Autodesk Inventor part; units mm, degrees
ref_plane "YZ Plane" through (0, 0, 0) normal (1, 0, 0) x (0, 1, 0)
ref_plane "XZ Plane" through (0, 0, 0) normal (0, 1, 0) x (-1, 0, 0)
ref_plane "XY Plane" through (0, 0, 0) normal (0, 0, 1) x (1, 0, 0)
sketch "Sketch1" plane through (0, 0, 0) normal (0, 1, 0) x (-1, 0, 0)
  circle A0 centre (0, 0) radius 90.805
  dimension "d0" = 181.61
extrude "Extrusion1" add sketch "Sketch1" along normal blind 6.35
sketch "Sketch2" plane through (0, 6.35, 0) normal (0, 1, 0) x (1, 0, 0)
  circle A0 centre (0, 0) radius 84.455
  dimension "d3" = 168.91
extrude "Extrusion2" add sketch "Sketch2" along normal blind 6.35
sketch "Sketch3" plane through (0, 12.7, 0) normal (0, 1, 0) x (1, 0, 0)
  circle A0 centre (0, 0) radius 93.98
  dimension "d6" = 187.96
extrude "Extrusion3" add sketch "Sketch3" along normal blind 6.35
sketch "Sketch4" plane through (0, 19.05, 0) normal (0, 1, 0) x (1, 0, 0)
  circle A0 centre (0, 0) radius 12.7
  circle A1 centre (-50.8, 0) radius 6.35
  dimension "d9" = 25.4
  dimension "d10" = 50.8
  dimension "d11" = 12.7
extrude "Extrusion4" cut sketch "Sketch4" against normal up to next
sketch "Sketch5" plane through (0, 19.05, 0) normal (0, 1, 0) x (1, 0, 0)
  circle A0 centre (0, 0) radius 93.98
  circle A1 centre (0, 0) radius 87.63
  dimension "d14" = 187.96
  dimension "d15" = 175.26
extrude "Extrusion5" add sketch "Sketch5" along normal blind 6.35
properties part number "thermal_barrier" material "Phenolic Resin"
Work out the finished part from the listing and answer in its coordinate system (mm). A direction names the side the tool comes from. Give positions to 0.01 mm unless a question says otherwise; leave off trailing zeros. Loops run counter-clockwise (first coordinate to the right, second up) from the corner with the lowest first, then second, coordinate; pieces in that order, holes last. Notation, with made-up numbers: (-13, 51.5) -> (12, 51.5) arc R20 ccw to (12, 69.5) -> close; hole circle Ø8 at (62.5, 84). An arc over 180 degrees is marked (long way). Use a Markdown table: item, result. Add a question column.
1) The part is cut by section B-B, the plane x = 0. Determine the outline of the cut face in (y, z) (3 decimals), plus the area to 3 significant figures.
2) The part is cut by section C-C, the plane z = -78. Determine the outline of the cut face in (x, y), plus the area to 3 significant figures.
3) Consider line 1 along X through (y, z) = (13.75, 0); line 2 along X through (y, z) = (22, 0); line 3 along Y through (x, z) = (79.5, -36). Determine where each line is inside the solid, lowest interval first.
4) For a pull along Y with two mould halves and no side action, classify faces 1 (the flat face through (-19, 0, 1)), 2 (the flat face through (-77, 25.4, -42.2)), 3 (the cylindrical face through (-2.75, 9.66, 12.4)), 4 (the cylindrical face through (38.971, 9.481, -74.926)) as +Y half, -Y half, draft (parallel to the pull), parting line (faces both ways), or undercut.
5) Each of these flat-tipped pins is pushed along its axis until it touches: P1, Ø10, axis at y = 17, z = -21, coming from the +X side; P2, Ø11.5, axis at x = -50.8, z = 0, coming from the -Y side; P3, Ø1.5, axis at x = -18, y = 3, coming from the +Z side; P4, Ø8, axis at x = -38, z = -17.5, coming from the +Y side. Where does it stop, or does it pass through?
6) Which of the six approach directions +Z, -Z, +X, -X, +Y, -Y give full straight-line access (tool end or side, diameter ignored) to faces 5 (the cylindrical face through (-86.61, 3.13, -27.28)), 6 (the flat face through (-60, 6.35, -60)), 7 (the cylindrical face through (-18.996, 22.181, -85.546))?
7) The part is cut by section D-D, the plane x = -50.8. Determine the outline of the cut face in (y, z), plus the area to 3 significant figures.
8) The part is cut by section A-A, the plane z = 0. Determine the outline of the cut face in (x, y) (3 decimals).
Reported:
| question | item | result |
|---|---|---|
| 1 | outline | (0, -90.805) -> (6.35, -90.805) -> (6.35, -84.455) -> (12.7, -84.455) -> (12.7, -93.98) -> (25.4, -93.98) -> (25.4, -87.63) -> (19.05, -87.63) -> (19.05, -12.7) -> (0, -12.7) -> close; (0, 12.7) -> (19.05, 12.7) -> (19.05, 87.63) -> (25.4, 87.63) -> (25.4, 93.98) -> (12.7, 93.98) -> (12.7, 84.455) -> (6.35, 84.455) -> (6.35, 90.805) -> (0, 90.805) -> close |
| 1 | area | 3,020 mm^2 |
| 2 | outline | (-52.42, 12.7) -> (-32.38, 12.7) -> (-32.38, 6.35) -> (-46.49, 6.35) -> (-46.49, 0) -> (46.49, 0) -> (46.49, 6.35) -> (32.38, 6.35) -> (32.38, 12.7) -> (52.42, 12.7) -> (52.42, 25.4) -> (39.94, 25.4) -> (39.94, 19.05) -> (-39.94, 19.05) -> (-39.94, 25.4) -> (-52.42, 25.4) -> close |
| 2 | area | 1,830 mm^2 |
| 3 | line 1 | x = -93.98 to -57.15, -44.45 to -12.7, 12.7 to 93.98 |
| 3 | line 2 | x = -93.98 to -87.63, 87.63 to 93.98 |
| 3 | line 3 | y = 0 to 6.35, 12.7 to 19.05 |
| 4 | face 1 | -Y half |
| 4 | face 2 | +Y half |
| 4 | face 3 | draft |
| 4 | face 4 | undercut |
| 5 | P1 | stops at x = 92.61 |
| 5 | P2 | passes through |
| 5 | P3 | stops at z = 89.15 |
| 5 | P4 | stops at y = 19.05 |
| 6 | face 5 | -Y |
| 6 | face 6 | none |
| 6 | face 7 | +Y |
| 7 | outline | (0, -75.27) -> (6.35, -75.27) -> (6.35, -67.47) -> (12.7, -67.47) -> (12.7, -79.07) -> (25.4, -79.07) -> (25.4, -71.4) -> (19.05, -71.4) -> (19.05, -6.35) -> (0, -6.35) -> close; (0, 6.35) -> (19.05, 6.35) -> (19.05, 71.4) -> (25.4, 71.4) -> (25.4, 79.07) -> (12.7, 79.07) -> (12.7, 67.47) -> (6.35, 67.47) -> (6.35, 75.27) -> (0, 75.27) -> close |
| 7 | area | 2,670 mm^2 |
| 8 | outline | (-93.98, 12.7) -> (-84.455, 12.7) -> (-84.455, 6.35) -> (-90.805, 6.35) -> (-90.805, 0) -> (-57.15, 0) -> (-57.15, 19.05) -> (-87.63, 19.05) -> (-87.63, 25.4) -> (-93.98, 25.4) -> close; (-44.45, 0) -> (-12.7, 0) -> (-12.7, 19.05) -> (-44.45, 19.05) -> close; (12.7, 0) -> (90.805, 0) -> (90.805, 6.35) -> (84.455, 6.35) -> (84.455, 12.7) -> (93.98, 12.7) -> (93.98, 25.4) -> (87.63, 25.4) -> (87.63, 19.05) -> (12.7, 19.05) -> close |
